Answer from the drawing. Dimensions are ordinates in mm from the lowest x, y and z of the part. A direction names the side the tool comes from. Give positions to 0.01 mm unless a question says otherwise; leave off trailing zeros. Write each loop counter-clockwise with the first axis right and the second up, starting at its lowest first coordinate (ties: lowest second). Pieces come first, ordered by that corner, then holes. Notation, with made-up numbers: (-20, -25.5) -> (13, -25.5) arc R11 ccw to (13, -5.5) -> close; hole circle Ø4 at (28.25, -15). An arc over 180 degrees is marked (long way). Write item = value, one per line.
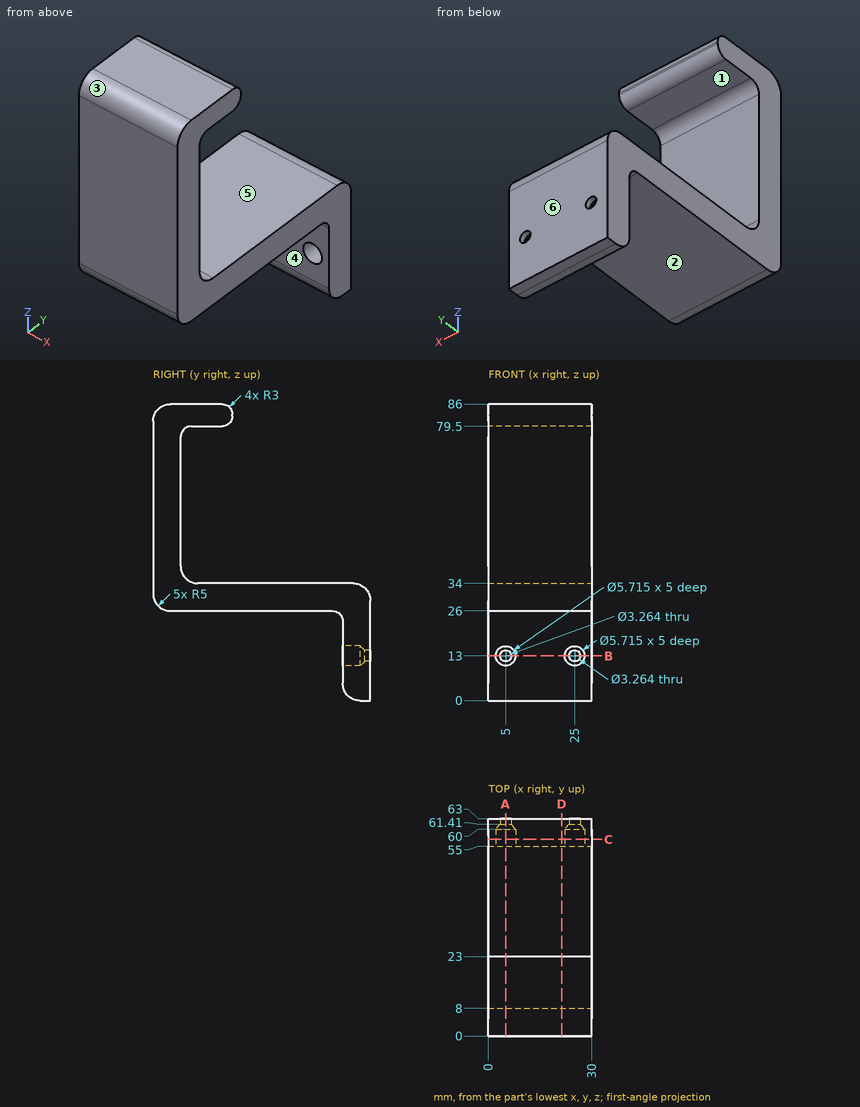
(1) The part is cut by section A-A on x = 5. Determine the outline of the cut face in (y, z).
Checks:
outline = (0, 31) arc R5 ccw to (5, 26) -> (52, 26) arc R3 cw to (55, 23) -> (55, 15.86) -> (60, 15.86) -> (61.41, 14.63) -> (63, 14.63) -> (63, 29) arc R5 ccw to (58, 34) -> (13, 34) arc R5 cw to (8, 39) -> (8, 76.5) arc R3 cw to (11, 79.5) -> (20, 79.5) arc R3 ccw to (23, 82.5) -> (23, 83) arc R3 ccw to (20, 86) -> (5, 86) arc R5 ccw to (0, 81) -> close; (55, 5) arc R5 ccw to (60, 0) -> (63, 0) -> (63, 11.37) -> (61.41, 11.37) -> (60, 10.14) -> (55, 10.14) -> close
(2) A tool of negligible diameter and unlimited length cuts with its end or side. For the marked faces 5 and 6, from which of +Z, -Z, +X, -X, +Y, -Y can it reach the whole face along a straight path? Write none if from no direction.
Checks:
face_5 = +X, -X, +Y
face_6 = +Z, -Z, +X, -X, +Y
(3) The part is cut by section B-B on z = 13. Determine the outline of the cut face in (x, y).
Checks:
outline = (0, 55) -> (2.14, 55) -> (2.14, 60) -> (3.37, 61.41) -> (3.37, 63) -> (0, 63) -> close; (6.63, 61.41) -> (7.86, 60) -> (7.86, 55) -> (22.14, 55) -> (22.14, 60) -> (23.37, 61.41) -> (23.37, 63) -> (6.63, 63) -> close; (26.63, 61.41) -> (27.86, 60) -> (27.86, 55) -> (30, 55) -> (30, 63) -> (26.63, 63) -> close
(4) For a pull along Z with two mould halves and no side action, classify the marked faces 1, 2, 3 and 4 as released by +Z, released by -Z, zero draft, split by the parting line, or undercut.
Checks:
face_1 = undercut
face_2 = released by -Z
face_3 = released by +Z
face_4 = zero draft
(5) The part is cut by section D-D on x = 21.25. Determine the outline of the cut face in (y, z).
Checks:
outline = (0, 31) arc R5 ccw to (5, 26) -> (52, 26) arc R3 cw to (55, 23) -> (55, 5) arc R5 ccw to (60, 0) -> (63, 0) -> (63, 29) arc R5 ccw to (58, 34) -> (13, 34) arc R5 cw to (8, 39) -> (8, 76.5) arc R3 cw to (11, 79.5) -> (20, 79.5) arc R3 ccw to (23, 82.5) -> (23, 83) arc R3 ccw to (20, 86) -> (5, 86) arc R5 ccw to (0, 81) -> close
(6) Consider L1, parallel to X at y = 58, z = 13; L2, parallel to X at y = 61.95, z = 13; L3, parallel to Y at x = 4, z = 5. Determine where each line is inside the solid, lowest interval first.
Checks:
L1 = 0 to 2.14, 7.86 to 22.14, 27.86 to 30
L2 = 0 to 3.37, 6.63 to 23.37, 26.63 to 30
L3 = 55 to 63
(7) The part is cut by section C-C on y = 57. Determine the outline of the cut face in (x, z) (1 decimal), plus the area to 3 significant figures.
Checks:
outline = (0, 1) -> (30, 1) -> (30, 34) -> (0, 34) -> close; hole circle Ø5.7 at (5, 13); hole circle Ø5.7 at (25, 13)
area = 939 mm²
(8) Given P1, Ø7.5, axis at x = 5, z = 13, coming from the -Y side; P2, Ø8, axis at x = 5, y = 44.5, coming from the +Z side; P3, Ø0.6, axis at x = 17, z = 82.5, coming from the +Y side; P4, Ø2, axis at x = 25, z = 13, coming from the -Y side, each flat-ended and moving along its own axis, determine where each tip first touches the part or whether it passes through.
Checks:
P1 = 55
P2 = 34
P3 = 23
P4 = through
